```python
from build123d import *

# Parameters (mm, degrees)
F1_DEPTH = 7
F2_R     = 2


with BuildPart() as f1:
    # F0 (on Top) → F1 (new body)
    with BuildSketch(Plane.XY):
        with BuildLine():
            ThreePointArc((-11.650635, -12.5), (-11.991377, -9.91181), (-12.990381, -7.5))
            ThreePointArc((-12.990381, -7.5), (-18.014847, -3.184365), (-24.634333, -2.955496))
            ThreePointArc((-24.634333, -2.955496), (-30.310889, -17.5), (-14.876701, -19.85621))
            ThreePointArc((-14.876701, -19.85621), (-12.492597, -16.516258), (-11.650635, -12.5))
        make_face()
        with BuildLine():
            ThreePointArc((-9.569581, -5.525), (-9.569581, 5.525), (0, 11.05))
            Line((0, 11.05), (0, 15))
            ThreePointArc((0, 15), (-6.249682, 17.193498), (-9.757631, 22.811706))
            ThreePointArc((-9.757631, 22.811706), (-12.167657, 7.025), (-24.634333, -2.955496))
            ThreePointArc((-24.634333, -2.955496), (-18.014847, -3.184365), (-12.990381, -7.5))
            Line((-12.990381, -7.5), (-9.569581, -5.525))
        make_face()
        with BuildLine():
            ThreePointArc((0, 11.05), (7.81353, 7.81353), (11.05, 0))
            ThreePointArc((11.05, 0), (10.67348, -2.85995), (9.569581, -5.525))
            Line((9.569581, -5.525), (12.990381, -7.5))
            ThreePointArc((12.990381, -7.5), (18.014847, -3.184365), (24.634333, -2.955496))
            ThreePointArc((24.634333, -2.955496), (12.167657, 7.025), (9.757631, 22.811706))
            ThreePointArc((9.757631, 22.811706), (6.249682, 17.193498), (0, 15))
            Line((0, 15), (0, 11.05))
        make_face()
        with BuildLine():
            ThreePointArc((-9.757631, 22.811706), (-6.249682, 17.193498), (0, 15))
            ThreePointArc((0, 15), (6.249682, 17.193498), (9.757631, 22.811706))
            ThreePointArc((9.757631, 22.811706), (9.939223, 23.899162), (10, 25))
            ThreePointArc((10, 25), (-1.100838, 34.939223), (-9.757631, 22.811706))
        make_face()
        with BuildLine():
            ThreePointArc((24.634333, -2.955496), (18.014847, -3.184365), (12.990381, -7.5))
            ThreePointArc((12.990381, -7.5), (11.765165, -14.009133), (14.876701, -19.85621))
            ThreePointArc((14.876701, -19.85621), (25.666893, -21.658039), (31.650635, -12.5))
            ThreePointArc((31.650635, -12.5), (29.707836, -6.577035), (24.634333, -2.955496))
        make_face()
        with BuildLine():
            Line((12.990381, -7.5), (9.569581, -5.525))
            ThreePointArc((9.569581, -5.525), (0, -11.05), (-9.569581, -5.525))
            Line((-9.569581, -5.525), (-12.990381, -7.5))
            ThreePointArc((-12.990381, -7.5), (-11.991377, -9.91181), (-11.650635, -12.5))
            ThreePointArc((-11.650635, -12.5), (-12.492597, -16.516258), (-14.876701, -19.85621))
            ThreePointArc((-14.876701, -19.85621), (0, -14.05), (14.876701, -19.85621))
            ThreePointArc((14.876701, -19.85621), (11.765165, -14.009133), (12.990381, -7.5))
        make_face()
    extrude(amount=F1_DEPTH)

    # F2
    f2_edges = [f1.edges().sort_by_distance(p)[0] for p in [
        (0, -14.05, 7),
        (0, -14.05, 0),
    ]]
    fillet(f2_edges, radius=F2_R)


solid = f1.part
```
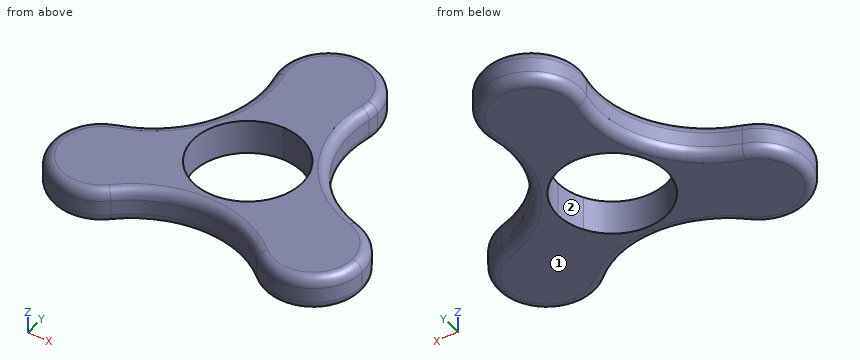
The listing builds one solid part. Answer for the finished solid, in the listing's coordinates (mm). Face numbers are marked on the shaded views. Give positions to 0.01 mm unless a question says otherwise; leave off trailing zeros. Loops run counter-clockwise (first coordinate to the right, second up) from the corner with the lowest first, then second, coordinate; pieces in that order, holes last. Notation, with made-up numbers: (72, 16.5) - (129, 16.5) arc R21 cw to (129, 55.5) - close; hole circle Ø2 at (25.5, -37.75). An arc over 180 degrees is marked (long way). Answer as CSV lines item,"result". Start each with the question number.
Item 1: Find the intervals of material crossed by line 1 (Y direction, x = -7.5, z = 2); line 2 (Y direction, x = 8.5, z = 5); line 3 (X direction, y = -16, z = 5.75), in increasing order. Write a range as from..to.
Item 2: The mould has two halves that part along X. Classify the marked faces 1 and 2: +X half, -X half, draft (parallel to the pull), parting line (faces both ways), or undercut.
Item 3: A cutting plane is placed at A-A on z = 5.75. Determine the outline of the cut face in (x, y) (3 decimals), then the cut area to 3 significant figures.
Item 4: Each of these flat-tipped pins is pushed along its axis until it touches: pin 1 (4 mm diameter, centred on x = -1, z = 1.5, fed in from -Y); pin 2 (3 mm diameter, centred on x = -9, y = -14, fed in from +Z); pin 3 (2 mm diameter, centred on x = 22.5, z = 6, fed in from +Y). Where does it stop, or does it pass through?
Found:
1,line 1,"y = -15.37..-8.11, 8.11..31.61"
1,line 2,"y = -15.76..-7.06, 7.06..30.27"
1,line 3,"x = -30.86..-9.4, 9.4..30.86"
2,face 1,"draft"
2,face 2,"undercut"
3,outline,"(-24.591, -3.095) arc R9.854 ccw (long way) to (-14.976, -19.749) arc R22.108 cw to (14.976, -19.749) arc R9.854 ccw (long way) to (24.591, -3.095) arc R22.108 cw to (9.615, 22.844) arc R9.854 ccw to (9.854, 25) arc R9.854 ccw (long way) to (-9.615, 22.844) arc R22.108 cw to start; hole (9.57, -5.525) arc R11.05 ccw to (11.05, 0) arc R11.05 ccw (long way) to start"
3,area,"1,390 mm^2"
4,pin 1,"stops at y = -14.25"
4,pin 2,"stops at z = 7"
4,pin 3,"stops at y = -1.84"
